Can you work these out from the model? Positions are in its coordinate system, mm. A direction names the side the tool comes from. Give positions to 0.01 mm unless a question says otherwise; leave off trailing zeros.
from build123d import *

# Parameters (mm, degrees)
SKETCH1_W                           = 9.525
SKETCH1_H                           = 15.875
BOSS_EXTRUDE1_DEPTH                 = 123.19
TAP_DRILL_FOR_10_32_TAP1_AT_2_COUNT = 2
TAP_DRILL_FOR_10_32_TAP1_AT_2_PITCH = 8.1788


with BuildPart() as part:
    # Sketch1 → Boss-Extrude1 (new, symmetric)
    with BuildSketch(Plane(origin=(0, 0, 0), x_dir=(0, 0, -1), z_dir=(1, 0, 0))):
        Rectangle(SKETCH1_W, SKETCH1_H)
    extrude(amount=BOSS_EXTRUDE1_DEPTH, both=True)

    # Sketch4 → Tap Drill for #10-32 Tap1 (revolve, cut)
    with BuildSketch(Plane(origin=(123.19, 4.0894, 0), x_dir=(0, 0, -1), z_dir=(0, 1, 0))):
        Polygon((0, 0), (0, 11.373317848), (2.0193, 10.16), (2.0193, 0), align=None)
    tap_drill_for_10_32_tap1 = revolve(axis=Axis((129.54, 4.0894, 0), (-1, 0, 0)), mode=Mode.SUBTRACT)

    # Tap Drill for #10-32 Tap1 at 2: Tap Drill for #10-32 Tap1 ×2
    with Locations(*[(0, -i * TAP_DRILL_FOR_10_32_TAP1_AT_2_PITCH, 0) for i in range(1, TAP_DRILL_FOR_10_32_TAP1_AT_2_COUNT)]):
        add(tap_drill_for_10_32_tap1, mode=Mode.SUBTRACT)

    # Mirror1: Tap Drill for #10-32 Tap1 across plane
    add(tap_drill_for_10_32_tap1.mirror(Plane(origin=(0, 0, 0), x_dir=(0, 0, 1), z_dir=(1, 0, 0))), mode=Mode.SUBTRACT)

    # Mirror1 copy 1 sketch → Mirror1 copy 1 (revolve, cut)
    with BuildSketch(Plane(origin=(-123.19, -4.0894, 0), x_dir=(0, 0, -1), z_dir=(0, 1, 0))):
        Polygon((0, 0), (0, -11.373317848), (2.0193, -10.16), (2.0193, 0), align=None)
    revolve(axis=Axis((-129.54, -4.0894, 0), (-1, 0, 0)), mode=Mode.SUBTRACT)


solid = part.part
(1) Will these pins go through, and if not, where does the flat tip stop? P1, Ø5.5, axis at y = -4.09, z = 0, coming from the +X side; P2, Ø3.5, axis at y = 4.09, z = 0, coming from the +X side; P3, Ø2.5, axis at y = 4.09, z = 0, coming from the -X side.
Returned:
P1: stops at x = 123.19
P2: stops at x = 112.87
P3: stops at x = -112.57
(2) If I drill on L1, parallel to Y at x = 118.5, z = 0; L2, parallel to X at y = -3, z = 1; L3, parallel to X at y = 4.5, z = -1.75, over which ranges is the centre line in solid material (lowest first)?
Returned:
L1: y = -7.94 to -6.11, -2.07 to 2.07, 6.11 to 7.94
L2: x = -112.71 to 112.71
L3: x = -112.9 to 112.9
(3) If we mould it in two halves opening along Z, with no side actions, what happens to faces 1 (the face through (-112.03, -4.44, 0.05)), 2 (the face through (-118.18, -2.12, 0.44)), 3 (the face through (2, 0, 4.762)), 4 (the face through (-123.19, 0, 0))? For each: +Z half, -Z half, draft (parallel to the pull), parting line (faces both ways), or undercut.
Returned:
face 1: undercut
face 2: undercut
face 3: +Z half
face 4: draft
(4) For faces 5 (the face through (2, -7.938, 0)), 6 (the face through (-118.181, 2.087, 0.263)), 7 (the face through (118.181, 2.087, 0.263)), which set-ups out of +Z, -Z, +X, -X, +Y, -Y let a thin tool reach every point of the face, with its end or its side?
Returned:
face 5: +Z, -Z, +X, -X, -Y
face 6: -X
face 7: +X
